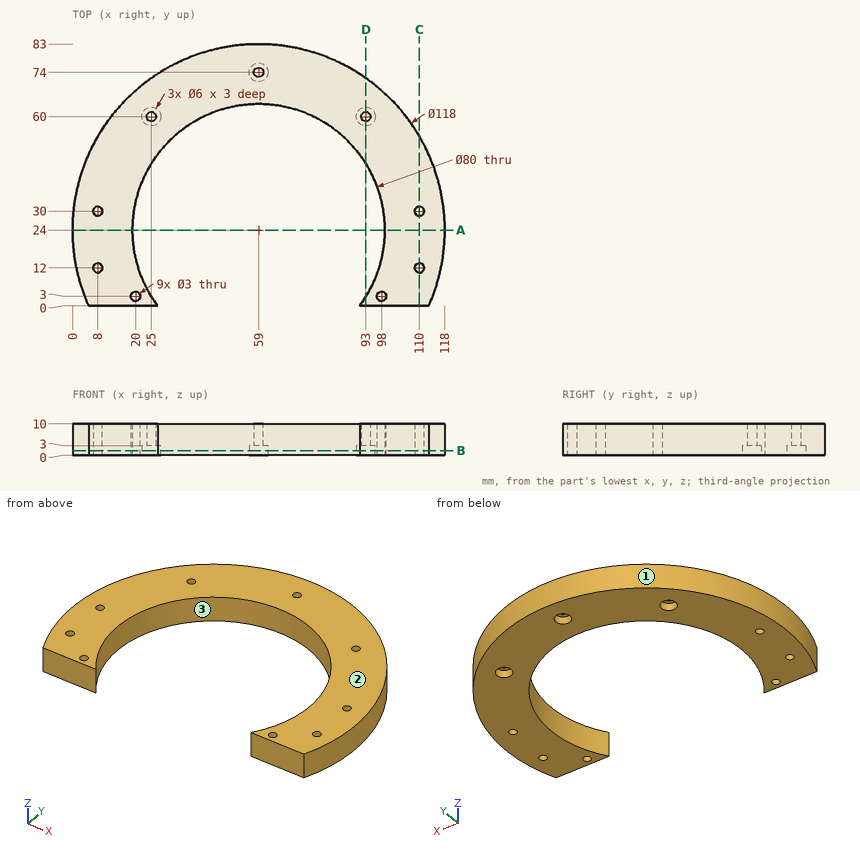
Geometry check sheet. Reference: drawing and pictorial views, mm from the part's lowest x, y, z. Coordinates: 2 decimals unless noted, no trailing zeros. Order: outer loops, then holes, each group sorted by start corner. A loop starts at its lowest first (then second) coordinate and runs counter-clockwise, first axis right, second up.
1. Sectioned sample at A-A, the plane y = 24. Record the cut outline in (x, z).
Results found:
outline: (0, 0) - (19, 0) - (19, 10) - (0, 10) - close; (99, 0) - (118, 0) - (118, 10) - (99, 10) - close
2. Sectioned sample at D-D, the plane x = 93. Record the cut outline in (y, z), and give its area (3 significant figures).
Results found:
outline: (0, 0) - (2.93, 0) - (2.93, 10) - (0, 10) - close; (45.07, 0) - (57, 0) - (57, 3) - (58.5, 3) - (58.5, 10) - (45.07, 10) - close; (61.5, 3) - (63, 3) - (63, 0) - (72.22, 0) - (72.22, 10) - (61.5, 10) - close
area: 262 mm2
3. Scan lines: line 1 (X direction, y = 24, z = 7.75); line 2 (Y direction, x = 110, z = 9); line 3 (Y direction, x = 59, z = 2). Record each from-to range of solid material in increasing order.
Results found:
line 1: x = 0 to 19, 99 to 118
line 2: y = 0 to 10.5, 13.5 to 28.5, 31.5 to 53.66
line 3: y = 64 to 71, 77 to 83
4. Go/stop test with flat-tipped pins: pin 1 Ø3 at (x, y) = (60, 75) entering from -Z; pin 2 Ø1 at (y, z) = (40, 7.5) entering from +X; pin 3 Ø5 at (x, z) = (75.5, 6) entering from -Y. Record where each tip stops, or that it passes through.
Results found:
pin 1: stops at z = 3
pin 2: stops at x = 115.93
pin 3: stops at y = 59.2
5. Sectioned sample at C-C, the plane x = 110. Record the cut outline in (y, z).
Results found:
outline: (0, 0) - (10.5, 0) - (10.5, 10) - (0, 10) - close; (13.5, 0) - (28.5, 0) - (28.5, 10) - (13.5, 10) - close; (31.5, 0) - (53.66, 0) - (53.66, 10) - (31.5, 10) - close
6. Release check for a two-part mould opening along X. For the marked faces 1, 2 and 3 record: +X half, -X half, draft (parallel to the pull), parting line (faces both ways), or undercut.
Results found:
face 1: parting line
face 2: draft
face 3: undercut
7. Sectioned sample at B-B, the plane z = 1.5. Give the number of separate pieces and of enclosed holes in the cut face, and give its area (3 significant figures).
Results found:
separate pieces: 1
enclosed holes: 9
area: 3,780 mm2
